For this review, take the finished solid that the model builds, in its own axes (mm). A direction names the side the tool comes from. Give positions to 0.01 mm unless a question says otherwise; leave off trailing zeros. Write each loop counter-clockwise with the first axis right and the second up, starting at its lowest first coordinate (ties: lowest second). Pieces come first, ordered by that corner, then holes.
from build123d import *

# Parameters (mm, degrees)
F0_W     = 32.5
F0_H     = 2
F1_DEPTH = 32.5
F2_R     = 1.5
F3_DEPTH = 3


with BuildPart() as f1:
    # F0 (on Top) → F1 (new body)
    with BuildSketch(Plane.XY):
        Rectangle(F0_W, F0_H)
    extrude(amount=F1_DEPTH)

    # F2 (on face) → F3 (join)
    with BuildSketch(Plane.XZ.offset(1)):
        with Locations((-5.18934, 11.06066)):
            Circle(F2_R)
        with Locations((7.68934, 23.93934)):
            Circle(F2_R)
    extrude(amount=F3_DEPTH)


solid = f1.part
(1) We need section B-B (y = -2.3). Write out the cut boundary in (x, z), and give its area (3 significant figures).
(2) We need section A-A (z = 23.5). Write out the cut boundary in (x, y), and give its area (3 significant figures).
(3) We need section C-C (x = 3). Write out the cut boundary in (y, z), and give its area (3 significant figures).
(4) For L1, parallel to Y at x = 10, z = 4; L2, parallel to X at y = -1.15, z = 24; L3, parallel to X at y = -2.65, z = 10, list the stretches that pass through material, from the lowest coordinate up.
(5) Clearance check with flat-ended pins moving along their axes: pin 1 Ø10 at (x, z) = (-5.5, 27) entering from -Y; pin 2 Ø3 at (y, z) = (-3, 9.5) entering from -X. State where each tip first meets the part, or that it passes through.
(6) Tool access review of faces 1 (the flat face through (0, 0, 32.5)), 2 (the cylindrical face through (8.38, -2.48, 22.61)): name each direction out of +Z, -Z, +X, -X, +Y, -Y from which nothing blocks a thin tool from reaching the whole face with its end or side.
(7) We need section D-D (z = 17). Write out the cut boundary in (x, y), and give its area (3 significant figures).
The answers:
1. outline: circle Ø3 at (-5.19, 11.06); circle Ø3 at (7.69, 23.94)
1. area: 14.1 mm2
2. outline: (-16.25, -1) - (6.26, -1) - (6.26, -4) - (9.12, -4) - (9.12, -1) - (16.25, -1) - (16.25, 1) - (-16.25, 1) - close
2. area: 73.6 mm2
3. outline: (-1, 0) - (1, 0) - (1, 32.5) - (-1, 32.5) - close
3. area: 65.0 mm2
4. L1: y = -1 to 1
4. L2: x = 6.19 to 9.19
4. L3: x = -6.25 to -4.13
5. pin 1: stops at y = -1
5. pin 2: stops at x = -6.69
6. face 1: +Z, +X, -X, +Y, -Y
6. face 2: -Y
7. outline: (-16.25, -1) - (16.25, -1) - (16.25, 1) - (-16.25, 1) - close
7. area: 65.0 mm2
